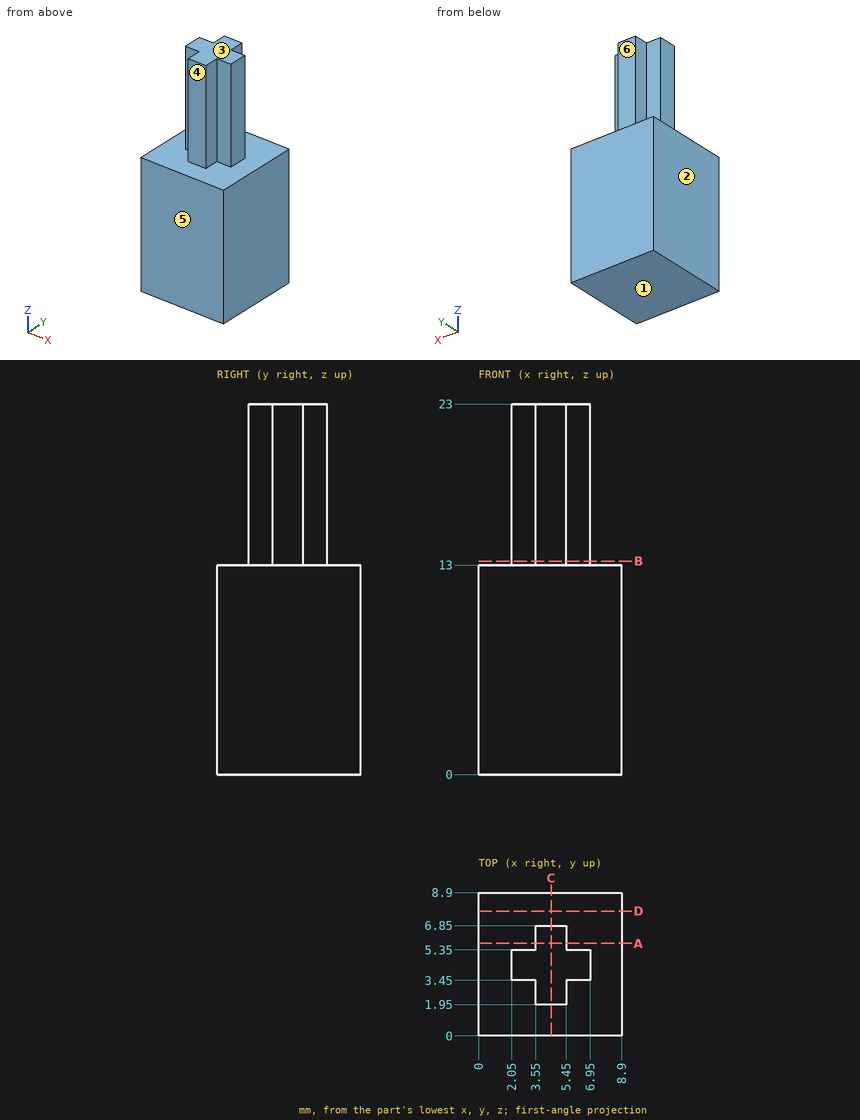
Here's the drawing with two shaded views (mm, measured from the low corner). I have some questions. A direction names the side the tool comes from. Give positions to 0.01 mm unless a question says otherwise; leave off trailing zeros. Write each loop counter-clockwise with the first axis right and the second up, starting at its lowest first coordinate (ties: lowest second). Pieces come first, ordered by that corner, then holes. Notation, with made-up numbers: (29, -23.5) -> (60, -23.5) arc R27 ccw to (60, -7.5) -> close; hole circle Ø2 at (7, 57.25). An arc over 180 degrees is marked (long way). Use one line per item in the form item = value. Start each with the question number.
1. Thinking about a two-plate mould opening in Z: for the marked faces 1, 2 and 3, which applies, +Z half, -Z half, draft (parallel to the pull), parting line (faces both ways), or undercut?
2. Imagine slicing it at A-A on y = 5.75. List the corners of the cut face in (x, z) for me.
3. Imagine slicing it at B-B on z = 13.25. List the corners of the cut face in (x, y) for me.
4. Imagine slicing it at D-D on y = 7.75. List the corners of the cut face in (x, z) for me.
5. On a 3-axis mill with a long thin cutter (end or side, diameter ignored), from which of +Z, -Z, +X, -X, +Y, -Y can I reach the whole of each face in a straight line? I mean the marked faces 4, 5 and 6. Say none if no direction works.
6. Imagine slicing it at C-C on x = 4.5. List the corners of the cut face in (y, z) for me, plus the area to 3 significant figures.
7. Will these pins go through, and if not, where does the flat tip stop? pin 1 Ø5 at (x, z) = (3, 18) entering from +Y; pin 2 Ø2 at (x, z) = (5, 16.5) entering from -Y; pin 3 Ø0.8 at (y, z) = (6.5, 17.5) entering from -X.
8. If I drill on L1, parallel to Z at x = 5.25, y = 8.75; L2, parallel to Y at x = 3.5, z = 15.25; L3, parallel to X at y = 4.5, z = 20, over which ranges is the centre line in solid material (lowest first)?
Entries:
q1.face_1 = -Z half
q1.face_2 = draft
q1.face_3 = +Z half
q2.outline = (0, 0) -> (8.9, 0) -> (8.9, 13) -> (5.45, 13) -> (5.45, 23) -> (3.55, 23) -> (3.55, 13) -> (0, 13) -> close
q3.outline = (2.05, 3.45) -> (3.55, 3.45) -> (3.55, 1.95) -> (5.45, 1.95) -> (5.45, 3.45) -> (6.95, 3.45) -> (6.95, 5.35) -> (5.45, 5.35) -> (5.45, 6.85) -> (3.55, 6.85) -> (3.55, 5.35) -> (2.05, 5.35) -> close
q4.outline = (0, 0) -> (8.9, 0) -> (8.9, 13) -> (0, 13) -> close
q5.face_4 = +Z, +X, -X, -Y
q5.face_5 = +Z, -Z, +X, -X, -Y
q5.face_6 = +Z, +X, -X, +Y
q6.outline = (0, 0) -> (8.9, 0) -> (8.9, 13) -> (6.85, 13) -> (6.85, 23) -> (1.95, 23) -> (1.95, 13) -> (0, 13) -> close
q6.area = 165 mm²
q7.pin_1 = 6.85
q7.pin_2 = 1.95
q7.pin_3 = 3.55
q8.L1 = 0 to 13
q8.L2 = 3.45 to 5.35
q8.L3 = 2.05 to 6.95
